from build123d import *

# Parameters (mm, degrees)
F1_W    = 5.1
F1_H    = 8
F1_W_2  = 1.2
F4_R    = 1
F5_SIZE = 0.2


with BuildPart() as f2:
    # F2: sweep along a path in F0
    with BuildLine(Plane.XZ) as f2_path:
        Line((0, 0), (0, -2))
    # F1 (on Top) → F2 (sweep)
    with BuildSketch(Plane.XY):
        Rectangle(F1_W, F1_H)
        with Locations((3.15, 0)):
            Rectangle(F1_W_2, F1_H)
        with Locations((-3.15, 0)):
            Rectangle(F1_W_2, F1_H)
    sweep(path=f2_path.line)

    # F3: sweep along a path in F0
    with BuildLine(Plane.XZ) as f3_path:
        Line((0, 0), (0, 1.9990060536))
    # F1 (on Top) → F3 (sweep)
    with BuildSketch(Plane.XY):
        with Locations((-3.15, 0)):
            Rectangle(F1_W_2, F1_H)
        with Locations((3.15, 0)):
            Rectangle(F1_W_2, F1_H)
    sweep(path=f3_path.line)

    # F4
    f4_edges = [f2.edges().sort_by_distance(p)[0] for p in [
        (-2.55, 4, 0.999503),
        (2.55, 4, 0.999503),
        (2.55, -4, 0.999503),
        (-2.55, -4, 0.999503),
    ]]
    fillet(f4_edges, radius=F4_R)

    # F5
    f5_edges = [f2.edges().sort_by_distance(p)[0] for p in [
        (0, -4, -2),
        (3.75, 0, -2),
        (0, 4, -2),
        (-3.75, 0, -2),
    ]]
    chamfer(f5_edges, length=F5_SIZE)


solid = f2.part
Build history of the part. All positions in model axes, mm. A direction names the side the tool comes from. Round coordinates to 2 decimals unless told otherwise and drop trailing zeros. Write each loop counter-clockwise with the first axis right and the second up, starting at its lowest first coordinate (ties: lowest second). Pieces come first, ordered by that corner, then holes. Notation, with made-up numbers: (54, -39) -> (66, -39) arc R25 cw to (66, -5) -> close; hole circle Ø7 at (21, 55). An arc over 180 degrees is marked (long way). Use one line per item in the form item = value.
Q1. Two-plate mould, pull along X, no slides. Class faces 1 (the flat face through (3.75, 0, 0)), 2 (the flat face through (0, -4, -1)), 3 (the flat face through (2.55, 0, 1)): released by +X, released by -X, zero draft, split by the parting line, or undercut.
Conclusion:
face_1 = released by +X
face_2 = zero draft
face_3 = undercut
Q2. Band-saw the part on A-A, the plane z = 0.45. Write the cut outline in (x, y).
Conclusion:
outline = (-3.75, -4) -> (-3.55, -4) arc R1 ccw to (-2.55, -3) -> (-2.55, 3) arc R1 ccw to (-3.55, 4) -> (-3.75, 4) -> close; (2.55, -3) arc R1 ccw to (3.55, -4) -> (3.75, -4) -> (3.75, 4) -> (3.55, 4) arc R1 ccw to (2.55, 3) -> close
Q3. Band-saw the part on D-D, the plane x = 1.5. Write the cut outline in (y, z).
Conclusion:
outline = (-4, -1.8) -> (-3.8, -2) -> (3.8, -2) -> (4, -1.8) -> (4, 0) -> (-4, 0) -> close
Q4. Tool access for faces 4 (the cylindrical face through (-2.835, 3.699, 1.013)), 5 (the cylindrical face through (2.835, -3.699, 1.013)), 6 (the flat face through (3, 0, 1.999)), 7 (the flat face through (-2.55, 0, 1)): list every direction of +Z, -Z, +X, -X, +Y, -Y with a clear straight run to the whole face (end or side of a thin tool).
Conclusion:
face_4 = +Z, +Y
face_5 = +Z, -Y
face_6 = +Z, +X, -X, +Y, -Y
face_7 = +Z, +Y, -Y
Q5. Drill centre lines: L1, parallel to X at y = -2.75, z = 1.35; L2, parallel to Z at x = -2, y = -2.75; L3, parallel to Y at x = 3.5, z = 0.2. Where is each one in solid material? Low to high.
Conclusion:
L1 = -3.75 to -2.55, 2.55 to 3.75
L2 = -2 to 0
L3 = -4 to 4
Q6. Band-saw the part on B-B, the plane y = 2.5. Write the cut outline in (x, z).
Conclusion:
outline = (-3.75, -1.8) -> (-3.55, -2) -> (3.55, -2) -> (3.75, -1.8) -> (3.75, 2) -> (2.55, 2) -> (2.55, 0) -> (-2.55, 0) -> (-2.55, 2) -> (-3.75, 2) -> close
Q7. Drop a flat-ended pin along its axis: P1, Ø3, axis at x = -1, y = 3, coming from the +Z side. Give the stop position or say it passes through.
Conclusion:
P1 = 0
Q8. Band-saw the part on C-C, the plane x = -2.75. Write the cut outline in (y, z).
Conclusion:
outline = (-4, -1.8) -> (-3.8, -2) -> (3.8, -2) -> (4, -1.8) -> (4, 0) -> (3.6, 0) -> (3.6, 2) -> (-3.6, 2) -> (-3.6, 0) -> (-4, 0) -> close
